from build123d import *

# Parameters (mm, degrees)
BOSS_EXTRUDE1_DEPTH      = 5.5
SKETCH2_R                = 1.65
CUT_EXTRUDE1_DEPTH       = 5.5
BOSS_EXTRUDE2_DEPTH      = 3
CUT_EXTRUDE2_DEPTH       = 2.75
SKETCH5_R                = 1.95
SKETCH5_R_2              = 1.35
SKETCH5_R_3              = 1.15
SKETCH5_R_4              = 2
CUT_EXTRUDE3_DEPTH       = 4.3
SKETCH7_R                = 1.95
SKETCH7_R_2              = 1.35
CUT_EXTRUDE4_DEPTH       = 3
CHAMFER1_SIZE            = 1
CUT_EXTRUDE5_DEPTH       = 2.75
SKETCH9_R                = 1.95
BOSS_EXTRUDE3_DEPTH      = 13.35
CUT_EXTRUDE6_START       = -8.8
SKETCH10_R               = 1
CUT_EXTRUDE6_DEPTH       = 8.8
SKETCH11_R               = 1.35
BOSS_EXTRUDE4_DEPTH      = 13.35
SKETCH12_R               = 1.15
BOSS_EXTRUDE5_DEPTH      = 6.9
SKETCH13_R               = 2
BOSS_EXTRUDE6_DEPTH      = 7.6
CUT_EXTRUDE7_START       = -3.3
SKETCH14_R               = 1
CUT_EXTRUDE7_DEPTH       = 3.3
BOSS_EXTRUDE7_DEPTH      = 3.1
BOSS_EXTRUDE7_DEPTH_BACK = 1.2
SKETCH15_R               = 1.65
SKETCH16_R               = 1
CUT_EXTRUDE8_DEPTH       = 3.1


with BuildPart() as part:
    # Sketch1 → Boss-Extrude1 (new body)
    with BuildSketch(Plane(origin=(0, 0, 0), x_dir=(1, 0, 0), z_dir=(0, 1, 0))):
        with BuildLine():
            Line((-7.755996733, 16.049992949), (-18.008818061, 22.554712546))
            ThreePointArc((-18.008818061, 22.554712546), (-25.669699487, 29.278547542), (-27.75, 19.3))
            Line((-27.75, 19.3), (-27.75, 8.1))
            Line((-27.75, 8.1), (-21.75, 2.8))
            Line((-21.75, 2.8), (-21.75, 0))
            Line((-21.75, 0), (21.75, 0))
            Line((21.75, 0), (21.75, 7))
            Line((21.75, 7), (18.25, 11))
            Line((18.25, 11), (-5.907756778, 15.263133549))
            ThreePointArc((-5.907756778, 15.263133549), (-6.75113203, 15.846223088), (-7.755996733, 16.049992949))
        make_face()
        with BuildLine():
            Line((-19.85, 18.630440726), (-10.05956754, 12.419075498))
            ThreePointArc((-10.05956754, 12.419075498), (-8.75757921, 11.15750472), (-6.94630287, 11.079964685))
            Line((-6.94630287, 11.079964685), (-0.119008465, 9.875148026))
            Line((-0.119008465, 9.875148026), (2.380991535, 6.875148026))
            Line((2.380991535, 6.875148026), (2.380991535, 1.3))
            Line((2.380991535, 1.3), (-12.151886792, 1.3))
            Line((-12.151886792, 1.3), (-19.85, 8.1))
            Line((-19.85, 8.1), (-19.85, 18.630440726))
        make_face(mode=Mode.SUBTRACT)
    extrude(amount=BOSS_EXTRUDE1_DEPTH)

    # Sketch2 → Cut-Extrude1 (cut)
    with BuildSketch(Plane(origin=(0, 5.5, 0), x_dir=(1, 0, 0), z_dir=(0, 1, 0))):
        with Locations(Location((-7.75, 13.5, 0), (0, 0, 270))):
            Circle(SKETCH2_R)
    extrude(amount=-CUT_EXTRUDE1_DEPTH, mode=Mode.SUBTRACT)

    # Sketch3 → Boss-Extrude2 (add)
    with BuildSketch(Plane(origin=(0, 5.5, 0), x_dir=(1, 0, 0), z_dir=(0, 1, 0))):
        with BuildLine():
            ThreePointArc((-27.75, 19.3), (-23.8, 17.782636193), (-19.85, 19.3))
            ThreePointArc((-19.85, 19.3), (-18.664735174, 20.777631), (-18.008818061, 22.554712546))
            ThreePointArc((-18.008818061, 22.554712546), (-17.927267525, 23.116055854), (-17.9, 23.682636193))
            ThreePointArc((-17.9, 23.682636193), (-26.198436991, 29.073137097), (-27.75, 19.3))
        make_face()
        with BuildLine():
            Line((-12.151886792, 1.3), (-19.85, 8.1))
            Line((-19.85, 8.1), (-19.85, 18.630440726))
            Line((-19.85, 18.630440726), (-19.85, 19.3))
            ThreePointArc((-19.85, 19.3), (-23.8, 17.782636193), (-27.75, 19.3))
            Line((-27.75, 19.3), (-27.75, 8.1))
            Line((-27.75, 8.1), (-21.75, 2.8))
            Line((-21.75, 2.8), (-21.75, 0))
            Line((-21.75, 0), (21.75, 0))
            Line((21.75, 0), (21.75, 1.3))
            Line((21.75, 1.3), (2.380991535, 1.3))
            Line((2.380991535, 1.3), (-12.151886792, 1.3))
        make_face()
    extrude(amount=BOSS_EXTRUDE2_DEPTH)

    # Sketch4 → Cut-Extrude2 (cut)
    with BuildSketch(Plane.XZ):
        with BuildLine():
            ThreePointArc((-27.75, -19.3), (-29.307610804, -25.798344876), (-23.8, -29.582636193))
            Line((-23.8, -29.582636193), (-23.8, -7.3))
            Line((-23.8, -7.3), (-26.844339623, -7.3))
            Line((-26.844339623, -7.3), (-27.75, -8.1))
            Line((-27.75, -8.1), (-27.75, -19.3))
        make_face()
    extrude(amount=-CUT_EXTRUDE2_DEPTH, mode=Mode.SUBTRACT)

    # Sketch5 → Cut-Extrude3 (cut)
    with BuildSketch(Plane.XZ):
        with Locations(Location((-23.8, -23.682636193, 0), (0, 0, 90))):
            Circle(SKETCH5_R)
        with Locations(Location((-23.8, -13.882636193, 0), (0, 0, 90))):
            Circle(SKETCH5_R_2)
        with Locations(Location((-20, -4.382636193, 0), (0, 0, 270))):
            Circle(SKETCH5_R_3)
        with Locations(Location((15.000589162, -5.5, 0), (0, 0, 270))):
            Circle(SKETCH5_R_4)
    extrude(amount=-CUT_EXTRUDE3_DEPTH, mode=Mode.SUBTRACT)

    # Sketch7 → Cut-Extrude4 (cut)
    with BuildSketch(Plane.XZ.offset(-4.3)):
        with Locations(Location((-23.8, -23.682636193, 0), (0, 0, 90))):
            Circle(SKETCH7_R)
        with Locations(Location((-23.8, -13.882636193, 0), (0, 0, 90))):
            Circle(SKETCH7_R_2)
    extrude(amount=-CUT_EXTRUDE4_DEPTH, mode=Mode.SUBTRACT)

    # Chamfer1
    chamfer1_edges = [part.edges().sort_by_distance(p)[0] for p in [
        (-23.8, 8.5, -29.582636193),
        (-27.75, 8.5, -13.7),
        (-24.75, 8.5, -5.45),
        (-21.75, 8.5, -1.4),
        (-19.85, 8.5, -13.7),
    ]]
    chamfer(chamfer1_edges, length=CHAMFER1_SIZE)

    # Sketch8 → Cut-Extrude5 (cut)
    with BuildSketch(Plane.XZ):
        with BuildLine():
            Line((-21.05, -7.3), (-23.8, -7.3))
            Line((-23.8, -7.3), (-23.8, -12.532636193))
            ThreePointArc((-23.8, -12.532636193), (-22.45, -13.882636193), (-23.8, -15.232636193))
            Line((-23.8, -15.232636193), (-23.8, -18.982636193))
            ThreePointArc((-23.8, -18.982636193), (-22.355013861, -19.210274953), (-21.05, -19.871140424))
            Line((-21.05, -19.871140424), (-21.05, -7.3))
        make_face()
        with BuildLine():
            ThreePointArc((-19.1, -23.682636193), (-19.615803542, -21.54195873), (-21.05, -19.871140424))
            ThreePointArc((-21.05, -19.871140424), (-22.355013861, -19.210274953), (-23.8, -18.982636193))
            Line((-23.8, -18.982636193), (-23.8, -21.732636193))
            ThreePointArc((-23.8, -21.732636193), (-21.85, -23.682636193), (-23.8, -25.632636193))
            Line((-23.8, -25.632636193), (-23.8, -28.382636193))
            ThreePointArc((-23.8, -28.382636193), (-20.476598128, -27.006038065), (-19.1, -23.682636193))
        make_face()
        with BuildLine():
            Line((-23.8, -21.732636193), (-23.8, -18.982636193))
            ThreePointArc((-23.8, -18.982636193), (-28.5, -23.682636193), (-23.8, -28.382636193))
            Line((-23.8, -28.382636193), (-23.8, -25.632636193))
            ThreePointArc((-23.8, -25.632636193), (-21.85, -23.682636193), (-23.8, -21.732636193))
        make_face()
    extrude(amount=-CUT_EXTRUDE5_DEPTH, mode=Mode.SUBTRACT)


with BuildPart() as body_2:
    # Mirror1: mirrored copy
    add(part.part.mirror(Plane.ZX))

    # Sketch9 → Boss-Extrude3 (add)
    with BuildSketch(Plane(origin=(0, -7.3, 0), x_dir=(1, 0, 0), z_dir=(0, 1, 0))):
        with Locations(Location((-23.8, 23.682636193, 0), (0, 0, 90))):
            Circle(SKETCH9_R)
    extrude(amount=BOSS_EXTRUDE3_DEPTH)

    # Sketch10 → Cut-Extrude6 (cut)
    with BuildSketch(Plane(origin=(0, 6.05, 0), x_dir=(1, 0, 0), z_dir=(0, 1, 0)).offset(CUT_EXTRUDE6_START)):
        with Locations(Location((-23.8, 23.682636193, 0), (0, 0, 270))):
            Circle(SKETCH10_R)
    extrude(amount=CUT_EXTRUDE6_DEPTH, mode=Mode.SUBTRACT)

    # Sketch11 → Boss-Extrude4 (add)
    with BuildSketch(Plane(origin=(0, -7.3, 0), x_dir=(1, 0, 0), z_dir=(0, 1, 0))):
        with Locations(Location((-23.8, 13.882636193, 0), (0, 0, 90))):
            Circle(SKETCH11_R)
    extrude(amount=BOSS_EXTRUDE4_DEPTH)

    # Sketch12 → Boss-Extrude5 (add)
    with BuildSketch(Plane(origin=(0, -4.3, 0), x_dir=(1, 0, 0), z_dir=(0, 1, 0))):
        with Locations(Location((-20, 4.382636193, 0), (0, 0, 90))):
            Circle(SKETCH12_R)
    extrude(amount=BOSS_EXTRUDE5_DEPTH)

    # Sketch13 → Boss-Extrude6 (add)
    with BuildSketch(Plane(origin=(0, -4.3, 0), x_dir=(1, 0, 0), z_dir=(0, 1, 0))):
        with Locations(Location((15.000589162, 5.5, 0), (0, 0, 90))):
            Circle(SKETCH13_R)
    extrude(amount=BOSS_EXTRUDE6_DEPTH)

    # Sketch14 → Cut-Extrude7 (cut)
    with BuildSketch(Plane(origin=(0, 3.3, 0), x_dir=(1, 0, 0), z_dir=(0, 1, 0)).offset(CUT_EXTRUDE7_START)):
        with Locations(Location((15.000589162, 5.5, 0), (0, 0, 270))):
            Circle(SKETCH14_R)
    extrude(amount=CUT_EXTRUDE7_DEPTH, mode=Mode.SUBTRACT)

    # Sketch15 → Boss-Extrude7 (add, two sides: drawn at the far end of the back side and taken through both)
    with BuildSketch(Plane(origin=(0, 0, 0), x_dir=(1, 0, 0), z_dir=(0, 1, 0)).offset(-BOSS_EXTRUDE7_DEPTH_BACK)):
        with Locations(Location((-7.75, 13.5, 0), (0, 0, 270))):
            Circle(SKETCH15_R)
    extrude(amount=BOSS_EXTRUDE7_DEPTH + BOSS_EXTRUDE7_DEPTH_BACK)

    # Sketch16 → Cut-Extrude8 (cut)
    with BuildSketch(Plane.XZ.offset(1.2)):
        with Locations(Location((-7.75, -13.5, 0), (0, 0, 270))):
            Circle(SKETCH16_R)
    extrude(amount=-CUT_EXTRUDE8_DEPTH, mode=Mode.SUBTRACT)


solid = body_2.part
Geometry check sheet. Reference: the model listing, model coordinates, mm. A direction names the side the tool comes from. Round coordinates to 2 decimals unless told otherwise and drop trailing zeros. Order: outer loops, then holes, each group sorted by start corner. A loop starts at its lowest first (then second) coordinate and runs counter-clockwise, first axis right, second up. Notation, with made-up numbers: M 83,20 L 115,20 A13 cw 115,26 Z; hole C 18.5,88 d1. An arc over 180 degrees is marked long. Write each question's results on one line, items separated by ' | '. Start each with the question number.
1. Draft check along Z on faces 1 (the face through (2.381, -3, -4)), 2 (the face through (-24, 6.05, -14)), 3 (the face through (-18.88, 1.28, -4.13)). Enter one of: pulls with the +Z half, pulls with the -Z half, needs draft (parallel to the pull), parting line crosses it, or undercut.
2. Cross-section at B-B on z = -13.5. Record the boundary of the cut face in (x, y), plus the area to 3 significant figures.
3. Set-up check for faces 4 (the face through (-25.733, 1.588, -23.429)), 5 (the face through (-23.8, -1, -29)), 6 (the face through (-9, -1.2, -14)): record each of +Z, -Z, +X, -X, +Y, -Y from which the full face is reachable in a straight line by a thin tool's end or side.
4. Cross-section at C-C on y = 4. Record the boundary of the cut face in (x, z).
5. Go/stop test with flat-tipped pins: P1, Ø3, axis at x = 12, z = -9.5, coming from the +Y side; P2, Ø0.7, axis at x = -19.5, z = -4.5, coming from the +Y side; P3, Ø2, axis at y = -1.5, z = -13.5, coming from the -X side. Record where each tip stops, or that it passes through.
6. Cross-section at A-A on y = -0.5. Record the boundary of the cut face in (x, z).
7. Material ranges on L1, parallel to X at y = 1.25, z = -23.75; L2, parallel to Y at x = 7, z = -2.5; L3, parallel to Z at x = 19.5, y = -7.5, recorded low to high. Write a range as from..to.
8. Cross-section at D-D on x = 6. Record the boundary of the cut face in (y, z), plus the area to 3 significant figures.
Resolved:
1) face 1: undercut | face 2: needs draft | face 3: parting line crosses it
2) outline: M -27.75,-7.5 L -26.75,-8.5 L -20.85,-8.5 L -19.85,-7.5 L -19.85,0 L -21.05,0 L -21.05,-2.75 L -22.51,-2.75 L -22.51,6.05 L -25.09,6.05 L -25.09,-2.75 L -27.75,-2.75 Z; M -11.76,-5.5 L -9.4,-5.5 L -9.4,-1.2 L -8.75,-1.2 L -8.75,1.9 L -6.75,1.9 L -6.75,-1.2 L -6.1,-1.2 L -6.1,-5.5 L 4.08,-5.5 L 4.08,0 L -6.1,0 L -6.1,3.1 L -9.4,3.1 L -9.4,0 L -11.76,0 Z | area: 148 mm2
3) face 4: +Y | face 5: -Z, -X, +Y | face 6: -Y
4) outline: C -23.8,-23.68 d3.9; C -23.8,-13.88 d2.7; hole C -23.8,-23.68 d2
5) P1: y = 0 | P2: y = 2.6 | P3: x = -25.15
6) outline: M -26.84,-7.3 L -21.05,-7.3 L -21.05,-19.87 A4.7 cw -23.8,-28.38 L -23.8,-29.58 A5.9 ccw -18.01,-22.55 L -7.76,-16.05 A2.55 ccw -5.91,-15.26 L 18.25,-11 L 21.75,-7 L 21.75,0 L -21.75,0 L -21.75,-2.8 Z; C -23.8,-23.68 d3.9; C -23.8,-13.88 d2.7; hole C -23.8,-23.68 d2; hole M -19.85,-18.63 L -10.06,-12.42 A2.55 cw -6.95,-11.08 L -0.12,-9.88 L 2.38,-6.88 L 2.38,-1.3 L -12.15,-1.3 L -19.85,-8.1 Z; hole C -7.75,-13.5 d2
7) L1: -25.75..-24.8, -22.8..-21.85 | L2: -5.5..0 | L3: -1.3..0
8) outline: M -8.5,-1.3 L -5.5,-1.3 L -5.5,-13.16 L 0,-13.16 L 0,0 L -8.5,0 Z | area: 76.3 mm2
